Design review of the part shown in the three views and the two pictorial views. Dimensions are in mm from the part's minimum x, y and z. Round coordinates to 2 decimals unless told otherwise and drop trailing zeros. Loops run counter-clockwise (first coordinate to the right, second up) from the corner with the lowest first, then second, coordinate; pieces in that order, holes last. Notation, with made-up numbers: (-32.5, 60.25) - (-14.5, 60.25) arc R11 ccw to (-14.5, 77.25) - close; hole circle Ø2 at (9, 10). An arc over 180 degrees is marked (long way). Return JSON: item names as keys, results as strings. Group by question number.
(1) The part is to be moulded in two halves that separate along Y. For the marked faces 1, 2 and 3, say which applies: pulls with the +Y half, pulls with the -Y half, needs draft (parallel to the pull), parting line crosses it, or undercut.
(2) Clearance check with flat-ended pins moving along their axes: pin 1 (2 mm diameter, centred on x = 84.5, z = 21.5, fed in from -Y); pin 2 (8 mm diameter, centred on x = 15, z = 44.5, fed in from +Y); pin 3 (2 mm diameter, centred on x = 70.5, z = 36, fed in from +Y). State where each tip first meets the part, or that it passes through.
(3) We need section D-D, the plane x = 26.25. Write out the cut boundary in (y, z).
(4) We need section B-B, the plane x = 50. Write out the cut boundary in (y, z).
(5) We need section C-C, the plane z = 30.5. Write out the cut boundary in (x, y) (3 decimals), and give its area (3 significant figures).
(6) We need section A-A, the plane y = 50. Write out the cut boundary in (x, z), and give its area (3 significant figures).
(7) Wall thickness on L1, parallel to Y at x = 46, z = 47.5; L2, parallel to Y at x = 25.5, z = 28 (1 decimal); L3, parallel to X at y = 53, z = 39 (1 decimal): over which ranges is each line inside the solid? List them lowest first. Write a range as [from, to].
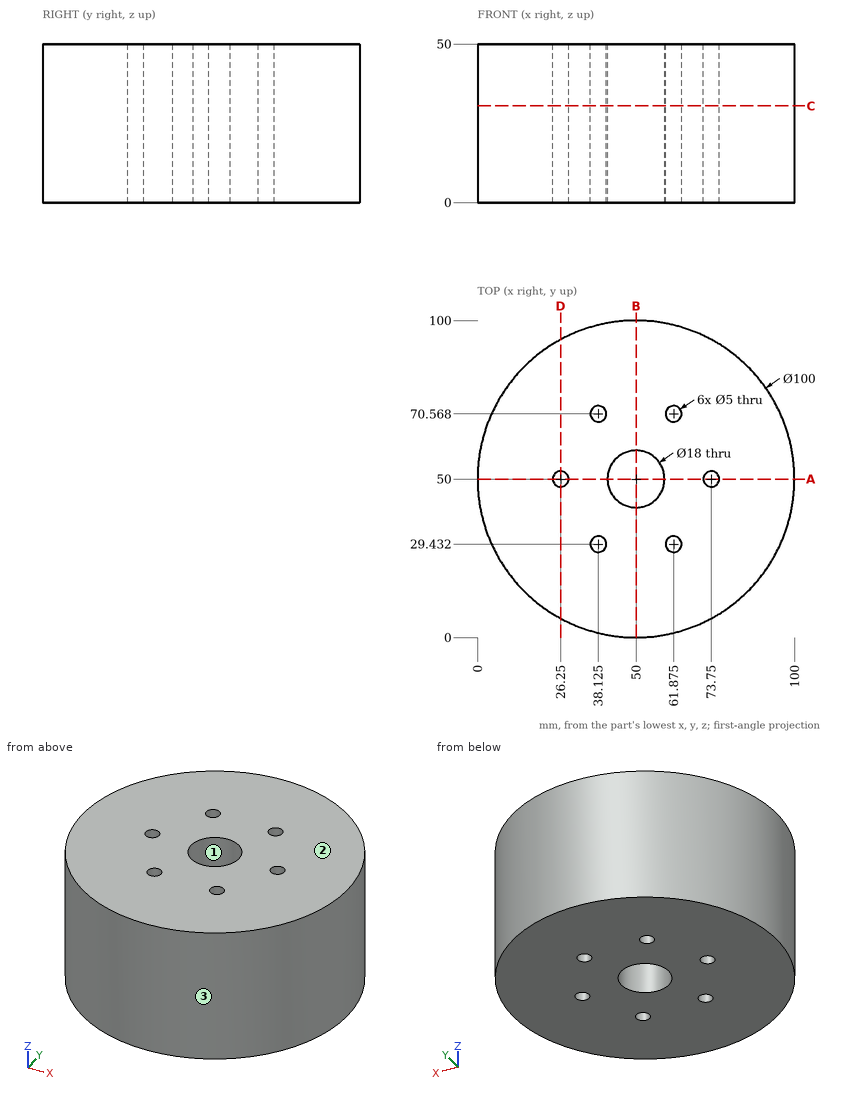
Solutions:
{
 "1": {"face 1": "undercut", "face 2": "needs draft", "face 3": "parting line crosses it"},
 "2": {"pin 1": "y = 12.88", "pin 2": "y = 89.23", "pin 3": "y = 96.04"},
 "3": {"outline": "(6, 0) - (47.5, 0) - (47.5, 50) - (6, 50) - close; (52.5, 0) - (94, 0) - (94, 50) - (52.5, 50) - close"},
 "4": {"outline": "(0, 0) - (41, 0) - (41, 50) - (0, 50) - close; (59, 0) - (100, 0) - (100, 50) - (59, 50) - close"},
 "5": {"outline": "circle Ø100 at (50, 50); hole circle Ø5 at (26.25, 50); hole circle Ø5 at (38.125, 29.432); hole circle Ø5 at (38.125, 70.568); hole circle Ø18 at (50, 50); hole circle Ø5 at (61.875, 29.432); hole circle Ø5 at (61.875, 70.568); hole circle Ø5 at (73.75, 50)", "area": "7,480 mm^2"},
 "6": {"outline": "(0, 0) - (23.75, 0) - (23.75, 50) - (0, 50) - close; (28.75, 0) - (41, 0) - (41, 50) - (28.75, 50) - close; (59, 0) - (71.25, 0) - (71.25, 50) - (59, 50) - close; (76.25, 0) - (100, 0) - (100, 50) - (76.25, 50) - close", "area": "3,600 mm^2"},
 "7": {"L1": "[0.16, 41.94], [58.06, 99.84]", "L2": "[6.4, 47.6], [52.4, 93.6]", "L3": "[0.1, 41.5], [58.5, 99.9]"}
}
